Geometry check sheet. Reference: the model listing, model coordinates, mm. Coordinates: 2 decimals unless noted, no trailing zeros. Order: outer loops, then holes, each group sorted by start corner. A loop starts at its lowest first (then second) coordinate and runs counter-clockwise, first axis right, second up. Notation, with made-up numbers: M 5,44 L 58,44 A28 cw 58,65 Z; hole C -34,19.5 d8. An arc over 180 degrees is marked long. One line per item, written item: value. Start each with the question number.
1) Sectioned sample at A-A, the plane z = -2. Enter the section's corners in (x, y), then the cut area to 3 significant figures.
2) Draft check along X on faces 1 (the conical face through (0.022, 9.042, -6.275)), 2 (the conical face through (7.78, 4.51, -0.06)), 3 (the cylindrical face through (-2.963, -3.864, -3.21)). Enter one of: pulls with the +X half, pulls with the -X half, needs draft (parallel to the pull), parting line crosses it, or undercut.
3) Go/stop test with flat-tipped pins: P1, Ø1.5, axis at x = 1.5, z = -5, coming from the +Y side; P2, Ø1, axis at x = -3.5, y = 2, coming from the +Z side. Record where each tip stops, or that it passes through.
4) Thickness scan on L1, parallel to X at y = 0, z = -2.15; L2, parallel to X at y = 4, z = -1.25; L3, parallel to Y at x = 0.75, z = -0.75. Record the ranges inside material, lowest first. Write a range as from..to.
Autodesk Inventor part; units mm, degrees
ref_plane "NUT_XY" through (0, 0, 0) normal (0, 0, 1) x (1, 0, 0)
ref_plane "NUT_YZ" through (0, 0, 0) normal (1, 0, 0) x (0, 1, 0)
ref_plane "NUT_ZX" through (0, 0, 0) normal (0, 1, 0) x (0, 0, 1)
sketch "Sketch_8" plane through (0, 0, 0) normal (1, 0, 0) x (0, 1, 0)
  line L0 (0, -6.35) -> (0, 0)
  line L1 (0, 0) -> (8.763, 0)
  line L2 (8.763, 0) -> (10.5156, -0.4696)
  line L3 (10.5156, -0.4696) -> (10.5156, -5.8804)
  line L4 (10.5156, -5.8804) -> (8.763, -6.35)
  line L5 (8.763, -6.35) -> (0, -6.35)
  line L6 (0, -6.35) -> (0, 0)
sketch "Sketch_10" plane through (0, 0, 0) normal (0, 0, 1) x (1, 0, 0)
  line L0 (-17.526, -17.526) -> (17.526, -17.526)
  line L1 (17.526, -17.526) -> (17.526, 17.526)
  line L2 (17.526, 17.526) -> (-17.526, 17.526)
  line L3 (-17.526, 17.526) -> (-17.526, -17.526)
  line L4 (-8.763, -5.0593) -> (0, -10.1186)
  line L5 (0, -10.1186) -> (8.763, -5.0593)
  line L6 (8.763, -5.0593) -> (8.763, 5.0593)
  line L7 (8.763, 5.0593) -> (0, 10.1186)
  line L8 (0, 10.1186) -> (-8.763, 5.0593)
  line L9 (-8.763, 5.0593) -> (-8.763, -5.0593)
revolve "Revolution1" add sketch "Sketch_8" angle 360 about axis through (0, 0, -6.35) along (0, 0, -1)
extrude "Extrusion1" cut sketch "Sketch_10" against normal blind 6.35
sketch "Sketch_11" plane through (0, 0, 0) normal (1, 0, 0) x (0, 1, 0)
  line L0 (0, -6.35) -> (0, 0)
  line L1 (0, 0) -> (5.5563, 0)
  line L2 (5.5563, 0) -> (4.8692, -0.6871)
  line L3 (4.8692, -0.6871) -> (4.8692, -5.6629)
  line L4 (4.8692, -5.6629) -> (5.5563, -6.35)
  line L5 (5.5563, -6.35) -> (0, -6.35)
  line L6 (0, -6.35) -> (0, 0)
revolve "Revolution2" cut sketch "Sketch_11" angle 360 about axis through (0, 0, -6.35) along (0, 0, -1)
thread "Thread1"
ref_plane "NUT_XY" through (0, 0, 0) normal (0, 0, 1) x (1, 0, 0)
ref_plane "NUT_YZ" through (0, 0, 0) normal (1, 0, 0) x (0, 1, 0)
ref_plane "NUT_ZX" through (0, 0, 0) normal (0, 1, 0) x (0, 0, 1)
ref_plane "a1_XY" through (-8.763, 8.763, 0) normal (0, 0, 1) x (1, 0, 0)
ref_plane "a1_YZ" through (-8.763, 8.763, 0) normal (1, 0, 0) x (0, 1, 0)
ref_plane "a1_ZX" through (-8.763, 8.763, 0) normal (0, 1, 0) x (0, 0, 1)
ref_plane "a2_XY" through (8.763, 8.763, 0) normal (0, 0, 1) x (1, 0, 0)
ref_plane "a2_YZ" through (8.763, 8.763, 0) normal (1, 0, 0) x (0, 1, 0)
ref_plane "a2_ZX" through (8.763, 8.763, 0) normal (0, 1, 0) x (0, 0, 1)
ref_plane "b1_XY" through (0, 8.763, 0) normal (1, 0, 0) x (0, 0, -1)
ref_plane "b1_YZ" through (0, 8.763, 0) normal (0, 0, -1) x (0, 1, 0)
ref_plane "b1_ZX" through (0, 8.763, 0) normal (0, 1, 0) x (1, 0, 0)
ref_plane "b2_XY" through (0, 8.763, -6.35) normal (1, 0, 0) x (0, 0, -1)
ref_plane "b2_YZ" through (0, 8.763, -6.35) normal (0, 0, -1) x (0, 1, 0)
ref_plane "b2_ZX" through (0, 8.763, -6.35) normal (0, 1, 0) x (1, 0, 0)
ref_plane "e_XY" through (0, 0, -6.35) normal (1, 0, 0) x (0, 0, -1)
ref_plane "e_YZ" through (0, 0, -6.35) normal (0, 0, -1) x (0, 1, 0)
ref_plane "e_ZX" through (0, 0, -6.35) normal (0, 1, 0) x (1, 0, 0)
ref_plane "ol1_XY" through (0, 0, -8.763) normal (0, 1, 0) x (1, 0, 0)
ref_plane "ol1_YZ" through (0, 0, -8.763) normal (1, 0, 0) x (0, 0, -1)
ref_plane "ol1_ZX" through (0, 0, -8.763) normal (0, 0, -1) x (0, 1, 0)
ref_plane "ol2_XY" through (6.35, 0, -8.763) normal (0, 1, 0) x (1, 0, 0)
ref_plane "ol2_YZ" through (6.35, 0, -8.763) normal (1, 0, 0) x (0, 0, -1)
ref_plane "ol2_ZX" through (6.35, 0, -8.763) normal (0, 0, -1) x (0, 1, 0)
ref_plane "th1_XY" through (0, 5.5563, -6.35) normal (1, 0, 0) x (0, 0, -1)
ref_plane "th1_YZ" through (0, 5.5563, -6.35) normal (0, 0, -1) x (0, 1, 0)
ref_plane "th1_ZX" through (0, 5.5563, -6.35) normal (0, 1, 0) x (1, 0, 0)
ref_plane "th2_XY" through (0, -5.5563, -6.35) normal (1, 0, 0) x (0, 0, -1)
ref_plane "th2_YZ" through (0, -5.5563, -6.35) normal (0, 0, -1) x (0, 1, 0)
ref_plane "th2_ZX" through (0, -5.5563, -6.35) normal (0, 1, 0) x (1, 0, 0)
properties part number "D-154"
Final values:
1. outline: M -8.76,-5.06 L 0,-10.12 L 8.76,-5.06 L 8.76,5.06 L 0,10.12 L -8.76,5.06 Z; hole C 0,0 d9.74
1. area: 192 mm^2
2. face 1: parting line crosses it
2. face 2: pulls with the +X half
2. face 3: undercut
3. P1: stops at y = 9.69
3. P2: passes through
4. L1: x = -8.76..-4.87, 4.87..8.76
4. L2: x = -8.76..-2.78, 2.78..8.76
4. L3: y = -9.69..-4.81, 4.81..9.69
